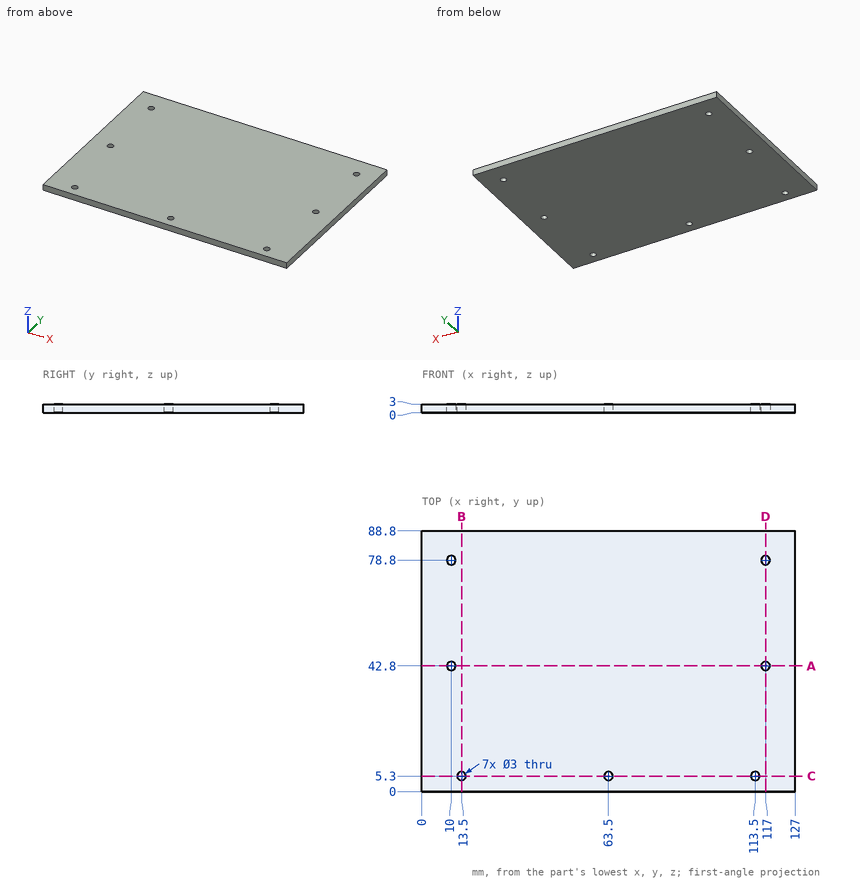
Design review of the part shown in the three views and the two pictorial views. Dimensions are in mm from the part's minimum x, y and z. Coordinates: 2 decimals unless noted, no trailing zeros. Order: outer loops, then holes, each group sorted by start corner. A loop starts at its lowest first (then second) coordinate and runs counter-clockwise, first axis right, second up.
1) Take a section at D-D, the plane x = 117. Give the boundary of the cut face in (y, z).
2) Wall thickness on line 1 along Y through (x, z) = (117, 0.75); line 2 along X through (y, z) = (5, 0.3); line 3 along X through (y, z) = (78.8, 1.6): over which ranges is each line inside the solid? List them lowest first.
3) Take a section at B-B, the plane x = 13.5. Give the boundary of the cut face in (y, z), and give its area (3 significant figures).
4) Take a section at A-A, the plane y = 42.8. Give the boundary of the cut face in (x, z).
5) Take a section at C-C, the plane y = 5.3. Give the boundary of the cut face in (x, z), and give its area (3 significant figures).
Returned:
1. outline: (0, 0) - (41.3, 0) - (41.3, 3) - (0, 3) - close; (44.3, 0) - (77.3, 0) - (77.3, 3) - (44.3, 3) - close; (80.3, 0) - (88.8, 0) - (88.8, 3) - (80.3, 3) - close
2. line 1: y = 0 to 41.3, 44.3 to 77.3, 80.3 to 88.8
2. line 2: x = 0 to 12.03, 14.97 to 62.03, 64.97 to 112.03, 114.97 to 127
2. line 3: x = 0 to 8.5, 11.5 to 115.5, 118.5 to 127
3. outline: (0, 0) - (3.8, 0) - (3.8, 3) - (0, 3) - close; (6.8, 0) - (88.8, 0) - (88.8, 3) - (6.8, 3) - close
3. area: 257 mm2
4. outline: (0, 0) - (8.5, 0) - (8.5, 3) - (0, 3) - close; (11.5, 0) - (115.5, 0) - (115.5, 3) - (11.5, 3) - close; (118.5, 0) - (127, 0) - (127, 3) - (118.5, 3) - close
5. outline: (0, 0) - (12, 0) - (12, 3) - (0, 3) - close; (15, 0) - (62, 0) - (62, 3) - (15, 3) - close; (65, 0) - (112, 0) - (112, 3) - (65, 3) - close; (115, 0) - (127, 0) - (127, 3) - (115, 3) - close
5. area: 354 mm2
